Check sheet for the modelled part. Datum: model origin and axes. Units: mm. A direction names the side the tool comes from. Give positions to 0.01 mm unless a question says otherwise; leave off trailing zeros. Order: outer loops, then holes, each group sorted by start corner. A loop starts at its lowest first (then second) coordinate and runs counter-clockwise, first axis right, second up.
```python
from build123d import *

# Parameters (mm, degrees)
ESTRUSIONE_ESTRUSIONE1_DEPTH = 16
RACCORDO1_R                  = 10
RACCORDO2_R                  = 20
SCHIZZO3_R                   = 1.5
TAGLIO_ESTRUSIONE1_DEPTH     = 16
SCHIZZO4_R                   = 2
TAGLIO_ESTRUSIONE2_DEPTH     = 1


with BuildPart() as part:
    # Schizzo1 → Estrusione-Estrusione1 (new body)
    with BuildSketch(Plane.XY):
        with BuildLine():
            ThreePointArc((3.856518615, 6.981794721), (0.004554283, 3.678491565), (3.5, 0))
            Line((3.5, 0), (43, 0))
            Line((43, 0), (43, 1))
            Line((43, 1), (11.5, 1))
            Line((11.5, 1), (11.5, 3))
            Line((11.5, 3), (32.826351822, 3))
            Line((32.826351822, 3), (43, 4.793888666))
            Line((43, 4.793888666), (42.826351822, 5.778696419))
            Line((42.826351822, 5.778696419), (32.826351822, 4.015426612))
            Line((32.826351822, 4.015426612), (3.856518615, 6.981794721))
        make_face()
    extrude(amount=ESTRUSIONE_ESTRUSIONE1_DEPTH)

    # Raccordo1
    raccordo1_edges = [part.edges().sort_by_distance(p)[0] for p in [
        (32.826351822, 4.015426612, 8),
    ]]
    fillet(raccordo1_edges, radius=RACCORDO1_R)

    # Raccordo2
    raccordo2_edges = [part.edges().sort_by_distance(p)[0] for p in [
        (32.826351822, 3, 8),
    ]]
    fillet(raccordo2_edges, radius=RACCORDO2_R)

    # Schizzo3 → Taglio-Estrusione1 (cut)
    with BuildSketch(Plane.XY.offset(16)):
        with Locations((10, 3.5)):
            Circle(SCHIZZO3_R)
    extrude(amount=-TAGLIO_ESTRUSIONE1_DEPTH, mode=Mode.SUBTRACT)

    # Schizzo4 → Taglio-Estrusione2 (cut)
    with BuildSketch(Plane.XZ):
        with Locations((40, 8)):
            Circle(SCHIZZO4_R)
        with Locations((15, 8)):
            Circle(SCHIZZO4_R)
    extrude(amount=-TAGLIO_ESTRUSIONE2_DEPTH, mode=Mode.SUBTRACT)


solid = part.part
```
(1) Release check for a two-part mould opening along Z. For faces 1 (the face through (38.526, 0.493, 9.352)), 2 (the face through (13.526, 0.493, 9.352)), 3 (the face through (43, 0.5, 7.9)), 4 (the face through (16, 4, 0)) record: released by +Z, released by -Z, zero draft, split by the parting line, or undercut.
(2) Go/stop test with flat-tipped pins: P1, Ø5, axis at x = 34, z = 10, coming from the +Y side; P2, Ø3, axis at y = 2, z = 11.5, coming from the +X side; P3, Ø5, axis at x = 24.5, z = 14, coming from the +Y side; P4, Ø1, axis at x = 32, z = 5, coming from the +Y side. Record where each tip stops, or that it passes through.
(3) Sectioned sample at B-B (z = 10.5). Enter the section's corners in (x, y).
(4) Sectioned sample at A-A (z = 8). Enter the section's corners in (x, y), plus the area to 3 significant figures.
(5) Tool access check on faces 5 (the face through (8.5, 3.57, 8.11)), 6 (the face through (38.72, 4.04, 7.89)), 7 (the face through (38.57, 5.03, 7.89)). Record the directions out of +Z, -Z, +X, -X, +Y, -Y that give a thin tool (end or side, any length) a straight path to the whole face; none if there is none.
(6) Sectioned sample at C-C (x = 36). Enter the section's corners in (y, z).
(7) Sectioned sample at D-D (x = 15). Enter the section's corners in (y, z), plus the area to 3 significant figures.
(8) Thickness scan on L1, parallel to Z at x = 15, y = 0.85; L2, parallel to Y at x = 41, z = 11.75; L3, parallel to Y at x = 28.5, z = 4.25. Record the ranges inside material, lowest first.
Values follow:
1. face 1: undercut
1. face 2: undercut
1. face 3: zero draft
1. face 4: released by -Z
2. P1: stops at y = 4.66
2. P2: stops at x = 43
2. P3: stops at y = 5.12
2. P4: stops at y = 4.15
3. outline: (3.5, 0) - (43, 0) - (43, 1) - (11.5, 1) - (11.5, 3) - (31.08, 3) arc R20 ccw to (34.55, 3.3) - (43, 4.79) - (42.83, 5.78) - (34.2, 4.26) arc R10 cw to (31.44, 4.16) - (3.86, 6.98) arc R3.5 ccw (long way) to start; hole circle Ø3 at (10, 3.5)
4. outline: (3.5, 0) - (13, 0) - (13, 1) - (11.5, 1) - (11.5, 3) - (31.08, 3) arc R20 ccw to (34.55, 3.3) - (43, 4.79) - (42.83, 5.78) - (34.2, 4.26) arc R10 cw to (31.44, 4.16) - (3.86, 6.98) arc R3.5 ccw (long way) to start; (17, 0) - (38, 0) - (38, 1) - (17, 1) - close; (42, 0) - (43, 0) - (43, 1) - (42, 1) - close; hole circle Ø3 at (10, 3.5)
4. area: 144 mm2
5. face 5: +Z, -Z
5. face 6: +Z, -Z, +X
5. face 7: +Z, -Z, +Y
6. outline: (0, 0) - (1, 0) - (1, 16) - (0, 16) - close; (3.56, 0) - (4.58, 0) - (4.58, 16) - (3.56, 16) - close
7. outline: (0, 0) - (1, 0) - (1, 6) - (0, 6) - close; (0, 10) - (1, 10) - (1, 16) - (0, 16) - close; (3, 0) - (5.84, 0) - (5.84, 16) - (3, 16) - close
7. area: 57.5 mm2
8. L1: z = 0 to 6, 10 to 16
8. L2: y = 0 to 1, 4.44 to 5.46
8. L3: y = 0 to 1, 3 to 4.46
